```python
from build123d import *

# Parameters (mm, degrees)
F0_R      = 30
F0_R_2    = 15
F1_DEPTH  = 20
F2_R      = 5
F3_DEPTH  = 50.4
F6_R      = 7.5
F7_DEPTH  = 10
F8_R      = 7.5
F9_DEPTH  = 10
F10_R     = 5
F11_DEPTH = 44.6
F13_R     = 7.5
F14_DEPTH = 10
F16_R     = 7.5
F17_DEPTH = 10


with BuildPart() as f1:
    # F0 (on Front) → F1 (new body, symmetric)
    with BuildSketch(Plane.XZ):
        Circle(F0_R)
        Circle(F0_R_2, mode=Mode.SUBTRACT)
    extrude(amount=F1_DEPTH, both=True)

    # F2 (on Top) → F3 (cut, symmetric)
    with BuildSketch(Plane.XY):
        Circle(F2_R)
    extrude(amount=F3_DEPTH, both=True, mode=Mode.SUBTRACT)

    # F6 (on offset) → F7 (cut)
    with BuildSketch(Plane.XY.offset(30)):
        Circle(F6_R)
    extrude(amount=-F7_DEPTH, mode=Mode.SUBTRACT)

    # F8 (on offset) → F9 (cut)
    with BuildSketch(Plane.XY.offset(-30)):
        Circle(F8_R)
    extrude(amount=F9_DEPTH, mode=Mode.SUBTRACT)

    # F10 (on Right) → F11 (cut, symmetric)
    with BuildSketch(Plane.YZ):
        Circle(F10_R)
    extrude(amount=F11_DEPTH, both=True, mode=Mode.SUBTRACT)

    # F13 (on offset) → F14 (cut)
    with BuildSketch(Plane.YZ.offset(30)):
        Circle(F13_R)
    extrude(amount=-F14_DEPTH, mode=Mode.SUBTRACT)

    # F16 (on offset) → F17 (cut)
    with BuildSketch(Plane.YZ.offset(-30)):
        Circle(F16_R)
    extrude(amount=F17_DEPTH, mode=Mode.SUBTRACT)


solid = f1.part
```
Part model, mm, in its own coordinate system. A direction names the side the tool comes from. Round coordinates to 2 decimals unless told otherwise and drop trailing zeros. Write each loop counter-clockwise with the first axis right and the second up, starting at its lowest first coordinate (ties: lowest second). Pieces come first, ordered by that corner, then holes. Notation, with made-up numbers: M -32,49 L 26,49 A18 cw 26,80 Z; hole C 41,34.5 d3. An arc over 180 degrees is marked long. Answer as CSV lines item,"result". Start each with the question number.
1) Mould opens along Y. For faces 1 (the face through (6, -20, 14)), 2 (the face through (20, 2, -5)), 3 (the face through (6, 20, 14)) say: +Y half, -Y half, draft (parallel to the pull), parting line (faces both ways), or undercut.
2) Which spindle directions (+Z, -Z, +X, -X, +Y, -Y) get a long thin tool onto all of the face, cutting with end or side? Do faces 4 (the face through (7.154, 2.253, 25.071)), 5 (the face through (6.93, -2.87, -25.07)), 6 (the face through (25.07, -7.493, 0.33)). Say none if no direction does.
3) Band-saw the part on D-D (x = -11.5). List the corners of the cut face in (y, z), then the cut area to 3 significant figures.
4) Band-saw the part on A-A (z = 0). List the corners of the cut face in (x, y).
5) Drop flat-ended pins along their axis: pin 1 (6 mm diameter, centred on x = 6, y = -5, fed in from +Z); pin 2 (11.5 mm diameter, centred on x = 0, y = 0, fed in from -Z); pin 3 (13 mm diameter, centred on y = 0, z = 0, fed in from -X). Give the stop position or say it passes through.
6) Drill centre lines: L1, parallel to Z at x = -2, y = -10; L2, parallel to X at y = -16, z = -3.5; L3, parallel to Z at x = 0, y = 6. Where is each one in solid material? Low to high.
7) Band-saw the part on B-B (x = 0). List the corners of the cut face in (y, z).
8) Band-saw the part on C-C (y = 0). Count the separate pieces of the cut face and the enclosed holes in it, then the cut area to 3 significant figures.
Worked out:
1,face 1,"-Y half"
1,face 2,"undercut"
1,face 3,"+Y half"
2,face 4,"+Z"
2,face 5,"-Z"
2,face 6,"+X"
3,outline,"M -20,-27.71 L 20,-27.71 L 20,-9.63 L -20,-9.63 Z; M -20,9.63 L 20,9.63 L 20,27.71 L -20,27.71 Z"
3,area,"1,450 mm²"
4,outline,"M -30,-20 L -15,-20 L -15,-5 L -20,-5 L -20,-7.5 L -30,-7.5 Z; M -30,7.5 L -20,7.5 L -20,5 L -15,5 L -15,20 L -30,20 Z; M 15,-20 L 30,-20 L 30,-7.5 L 20,-7.5 L 20,-5 L 15,-5 Z; M 15,5 L 20,5 L 20,7.5 L 30,7.5 L 30,20 L 15,20 Z"
5,pin 1,"z = 29.8"
5,pin 2,"z = -20"
5,pin 3,"x = -20"
6,L1,"-29.93 to -14.87, 14.87 to 29.93"
6,L2,"-29.8 to -14.59, 14.59 to 29.8"
6,L3,"-20 to -15, 15 to 20"
7,outline,"M -20,-30 L -7.5,-30 L -7.5,-20 L -5,-20 L -5,-15 L -20,-15 Z; M -20,15 L -5,15 L -5,20 L -7.5,20 L -7.5,30 L -20,30 Z; M 5,-20 L 7.5,-20 L 7.5,-30 L 20,-30 L 20,-15 L 5,-15 Z; M 5,15 L 20,15 L 20,30 L 7.5,30 L 7.5,20 L 5,20 Z"
8,separate pieces,"4"
8,enclosed holes,"0"
8,area,"1,330 mm²"
